Read the model definition and answer for the solid it produces. Units are mm, in the model's axes. Face numbers are marked on the shaded views. A direction names the side the tool comes from. Coordinates: 2 decimals unless noted, no trailing zeros. Order: outer loops, then holes, each group sorted by start corner. A loop starts at its lowest first (then second) coordinate and runs counter-clockwise, first axis right, second up. Notation, with made-up numbers: (57.5, 31) -> (87.5, 31) arc R13 cw to (87.5, 36) -> close; hole circle Ø6 at (39, 84). An arc over 180 degrees is marked (long way). Answer in a Markdown table with one row per item.
from build123d import *

# Parameters (mm, degrees)
SKETCH1_R           = 11
BOSS_EXTRUDE1_DEPTH = 6.5
SKETCH2_R           = 9
BOSS_EXTRUDE2_DEPTH = 5.5
SKETCH3_R           = 3
CUT_EXTRUDE1_DEPTH  = 15.5
SKETCH4_R           = 1.6
CUT_EXTRUDE2_DEPTH  = 15.5
CIRPATTERN1_COUNT   = 3


with BuildPart() as part:
    # Sketch1 → Boss-Extrude1 (new body)
    with BuildSketch(Plane(origin=(0, 0, 0), x_dir=(1, 0, 0), z_dir=(0, 1, 0))):
        with Locations(Location((-22.120080678, 12.823767702, 0), (0, 0, 90))):
            Circle(SKETCH1_R)
    extrude(amount=BOSS_EXTRUDE1_DEPTH)

    # Sketch2 → Boss-Extrude2 (add)
    with BuildSketch(Plane(origin=(0, 6.5, 0), x_dir=(1, 0, 0), z_dir=(0, 1, 0))):
        with Locations(Location((-22.120080678, 12.823767702, 0), (0, 0, 270))):
            Circle(SKETCH2_R)
    extrude(amount=BOSS_EXTRUDE2_DEPTH)

    # Sketch3 → Cut-Extrude1 (cut)
    with BuildSketch(Plane(origin=(0, 12, 0), x_dir=(1, 0, 0), z_dir=(0, 1, 0))):
        with Locations(Location((-22.120080678, 12.823767702, 0), (0, 0, 270))):
            Circle(SKETCH3_R)
    extrude(amount=-CUT_EXTRUDE1_DEPTH, mode=Mode.SUBTRACT)

    # Sketch4 → Cut-Extrude2 (cut)
    with BuildSketch(Plane(origin=(0, 12, 0), x_dir=(1, 0, 0), z_dir=(0, 1, 0))):
        with Locations(Location((-15.920080678, 12.823767702, 0), (0, 0, 270))):
            Circle(SKETCH4_R)
    cut_extrude2 = extrude(amount=-CUT_EXTRUDE2_DEPTH, mode=Mode.SUBTRACT)

    # CirPattern1: Cut-Extrude2 ×3 about axis
    cirpattern1_axis = Axis((-22.120080678, 0, -12.823767702), (0, 1, 0))
    for i in range(1, CIRPATTERN1_COUNT):
        add(cut_extrude2.rotate(cirpattern1_axis, i * 360 / CIRPATTERN1_COUNT), mode=Mode.SUBTRACT)


solid = part.part
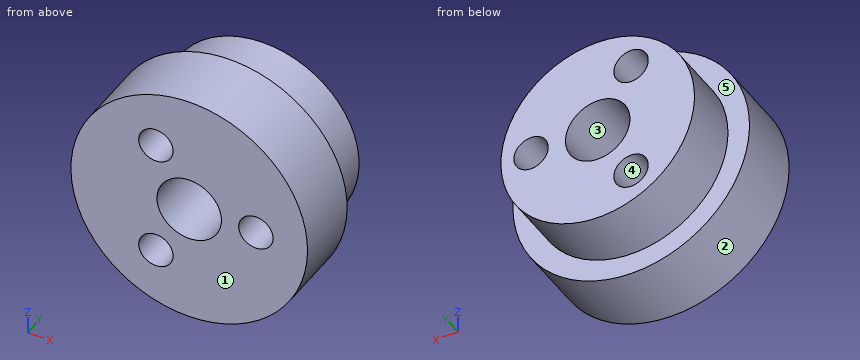
Q1. The part is cut by section D-D (z = -20.5). Write down the section's boundary in (x, y), then the cut area to 3 significant figures.
Outcome:
| item | result |
|---|---|
| outline | (-30, 0) -> (-14.24, 0) -> (-14.24, 6.5) -> (-17.42, 6.5) -> (-17.42, 12) -> (-26.82, 12) -> (-26.82, 6.5) -> (-30, 6.5) -> close |
| area | 154 mm² |
Q2. Given pin 1 (5 mm diameter, centred on x = -28, y = 10, fed in from +Z); pin 2 (1.5 mm diameter, centred on x = -19.5, y = 4.5, fed in from -Z); pin 3 (5 mm diameter, centred on x = -25.22, z = -7.45, fed in from +Y); pin 4 (1.5 mm diameter, centred on y = 6, z = -15, fed in from -X), each flat-ended and moving along its own axis, determine where each tip first touches the part or whether it passes through.
Outcome:
| item | result |
|---|---|
| pin 1 | z = -4.48 |
| pin 2 | z = -23.66 |
| pin 3 | y = 12 |
| pin 4 | x = -33.03 |
Q3. For the marked faces 4 and 5, determine the directions among +Z, -Z, +X, -X, +Y, -Y from which every point of the face is accessible in a straight line to the end or side of a thin tool.
Outcome:
| item | result |
|---|---|
| face 4 | +Y, -Y |
| face 5 | +Y |
Q4. The part is cut by section C-C (x = -28.25). Write down the section's boundary in (y, z).
Outcome:
| item | result |
|---|---|
| outline | (0, -21.96) -> (6.5, -21.96) -> (6.5, -19.41) -> (12, -19.41) -> (12, -6.23) -> (6.5, -6.23) -> (6.5, -3.69) -> (0, -3.69) -> close |
Q5. The part is cut by section B-B (y = 2.75). Write down the section's boundary in (x, z).
Outcome:
| item | result |
|---|---|
| outline | circle Ø22 at (-22.12, -12.82); hole circle Ø3.2 at (-25.22, -18.19); hole circle Ø3.2 at (-25.22, -7.45); hole circle Ø6 at (-22.12, -12.82); hole circle Ø3.2 at (-15.92, -12.82) |
Q6. Consider line 1 (Z direction, x = -24, y = 9.5); line 2 (X direction, y = 2.75, z = -13.75); line 3 (X direction, y = 3.75, z = -6). Determine where each line is inside the solid, lowest interval first.
Outcome:
| item | result |
|---|---|
| line 1 | -21.63 to -19.23, -17.16 to -15.16, -10.49 to -8.49, -6.42 to -4.02 |
| line 2 | -33.08 to -24.97, -19.27 to -17.22, -14.62 to -11.16 |
| line 3 | -30.75 to -25.89, -24.55 to -13.49 |
Q7. The part is cut by section A-A (x = -22.5). Write down the section's boundary in (y, z), then the cut area to 3 significant figures.
Outcome:
| item | result |
|---|---|
| outline | (0, -23.82) -> (6.5, -23.82) -> (6.5, -21.82) -> (12, -21.82) -> (12, -15.8) -> (0, -15.8) -> close; (0, -9.85) -> (12, -9.85) -> (12, -3.83) -> (6.5, -3.83) -> (6.5, -1.83) -> (0, -1.83) -> close |
| area | 170 mm² |
Q8. For a pull along X with two mould halves and no side action, classify the marked faces 1, 2 and 3 as pulls with the +X half, pulls with the -X half, needs draft (parallel to the pull), parting line crosses it, or undercut.
Outcome:
| item | result |
|---|---|
| face 1 | needs draft |
| face 2 | parting line crosses it |
| face 3 | undercut |
